Can you work these out from the model? Positions are in its coordinate system, mm. A direction names the side the tool comes from. Give positions to 0.01 mm unless a question says otherwise; leave off trailing zeros. Loops run counter-clockwise (first coordinate to the right, second up) from the corner with the lowest first, then second, coordinate; pieces in that order, holes last. Notation, with made-up numbers: (47, -12) -> (76, -12) arc R11 cw to (76, -5) -> close; hole circle Ø10 at (-29.75, 84). An arc over 180 degrees is marked (long way). One line per question, with ' | ' between items.
from build123d import *

# Parameters (mm, degrees)
SKETCH1_R           = 1.4
BOSS_EXTRUDE1_DEPTH = 11.25
SKETCH2_R           = 1.46
BOSS_EXTRUDE2_DEPTH = 3.5
SKETCH3_R           = 1.875
BOSS_EXTRUDE3_DEPTH = 1.21


with BuildPart() as part:
    # Sketch1 → Boss-Extrude1 (new body)
    with BuildSketch(Plane(origin=(0, 0, 0), x_dir=(1, 0, 0), z_dir=(0, 1, 0))):
        Circle(SKETCH1_R)
    extrude(amount=BOSS_EXTRUDE1_DEPTH)

    # Sketch2 → Boss-Extrude2 (add)
    with BuildSketch(Plane(origin=(0, 11.25, 0), x_dir=(1, 0, 0), z_dir=(0, 1, 0))):
        Circle(SKETCH2_R)
    extrude(amount=-BOSS_EXTRUDE2_DEPTH)

    # Sketch3 → Boss-Extrude3 (add)
    with BuildSketch(Plane.XZ.offset(-7.75)):
        Circle(SKETCH3_R)
    extrude(amount=-BOSS_EXTRUDE3_DEPTH)


solid = part.part
Q1. If we section it at D-D (y = 5.25): Write out the boundary of the cut face in (x, z), plus the area to 3 significant figures.
Entries:
outline: circle Ø2.8 at (0, 0) | area: 6.16 mm²
Q2. For pin 1 Ø1.5 at (y, z) = (10, -0.5) entering from -X, with a flat end and sliding along its axis, tell me the tip position at first contact or that it passes through.
Entries:
pin 1: x = -1.46
Q3. On a 3-axis mill with a long thin cutter (end or side, diameter ignored), from which of +Z, -Z, +X, -X, +Y, -Y can I reach the whole of each face in a straight line? I mean faces 1 (the face through (-1.873, 8.347, 0.082)), 2 (the face through (1.393, 10.121, -0.439)), 3 (the face through (-1.4, 3.82, -0.06)). Say none if no direction works.
Entries:
face 1: +Y, -Y | face 2: +Y | face 3: -Y
Q4. If we section it at C-C (y = 9.25): Write out the boundary of the cut face in (x, z), plus the area to 3 significant figures.
Entries:
outline: circle Ø2.92 at (0, 0) | area: 6.70 mm²
Q5. If I drill on probe 1 along Y at (x, z) = (0.7, 1.35); probe 2 along X at (y, z) = (7.5, 0.05); probe 3 along Z at (x, y) = (-0.05, 10), over which ranges is the centre line in solid material (lowest first)? Write a range as from..to.
Entries:
probe 1: 7.75..8.96 | probe 2: -1.4..1.4 | probe 3: -1.46..1.46
Q6. If we section it at B-B (z = 0): Write out the boundary of the cut face in (x, y) (3 decimals).
Entries:
outline: (-1.875, 7.75) -> (-1.4, 7.75) -> (-1.4, 0) -> (1.4, 0) -> (1.4, 7.75) -> (1.875, 7.75) -> (1.875, 8.96) -> (1.46, 8.96) -> (1.46, 11.25) -> (-1.46, 11.25) -> (-1.46, 8.96) -> (-1.875, 8.96) -> close
Q7. If we section it at A-A (x = 0): Write out the boundary of the cut face in (y, z) (3 decimals), plus the area to 3 significant figures.
Entries:
outline: (0, -1.4) -> (7.75, -1.4) -> (7.75, -1.875) -> (8.96, -1.875) -> (8.96, -1.46) -> (11.25, -1.46) -> (11.25, 1.46) -> (8.96, 1.46) -> (8.96, 1.875) -> (7.75, 1.875) -> (7.75, 1.4) -> (0, 1.4) -> close | area: 32.9 mm²
